Geometry: final body of the model. Coordinates: model frame, mm. A direction names the side the tool comes from. Give positions to 0.01 mm unless a question says otherwise; leave off trailing zeros. Order: outer loops, then holes, each group sorted by start corner. A loop starts at its lowest first (then second) coordinate and runs counter-clockwise, first axis right, second up. Notation, with made-up numbers: M 75.5,-40 L 130.5,-40 A24 ccw 130.5,-12 Z; hole C 54,79 d3. An arc over 180 degrees is marked long. Use CSV: the item, a comma, the result in double quotes.
```python
from build123d import *

# Parameters (mm, degrees)
PAD_DEPTH    = 12
SKETCH001_W  = 160
SKETCH001_H  = 100
PAD001_DEPTH = 10
SKETCH002_R  = 2
POCKET_DEPTH = 22.001


with BuildPart() as part:
    # Sketch → Pad (new body)
    with BuildSketch(Plane.XY):
        Polygon((-50, 340), (50, 340), (50, 100), (80, 100), (80, 0), (50, 0), (50, -11), (-50, -11), (-50, 0), (-80, 0), (-80, 100), (-50, 100), align=None)
    extrude(amount=PAD_DEPTH)

    # Sketch001 (on Face14 of Pad) → Pad001 (join)
    with BuildSketch(Plane.XY.offset(12)):
        with Locations((0, 50)):
            Rectangle(SKETCH001_W, SKETCH001_H)
    extrude(amount=PAD001_DEPTH)

    # Sketch002 (on Face18 of Pad001) → Pocket (cut, through all)
    with BuildSketch(Plane.XY.offset(22)):
        with Locations((-69.908607, 88.239746)):
            Circle(SKETCH002_R)
        with Locations((69.908607, 88.239746)):
            Circle(SKETCH002_R)
        with Locations((69.908607, 10.851752)):
            Circle(SKETCH002_R)
        with Locations((-69.908607, 10.851752)):
            Circle(SKETCH002_R)
    extrude(amount=-POCKET_DEPTH, mode=Mode.SUBTRACT)


solid = part.part
```
1. Section A-A, the plane x = -46. Return the cut outline in (y, z), plus the area to 3 significant figures.
Answer:
outline,"M -11,0 L 340,0 L 340,12 L 100,12 L 100,22 L 0,22 L 0,12 L -11,12 Z"
area,"5,210 mm2"
2. Section B-B, the plane z = 3.25. Return the cut outline in (x, y), plus the area to 3 significant figures.
Answer:
outline,"M -80,0 L -50,0 L -50,-11 L 50,-11 L 50,0 L 80,0 L 80,100 L 50,100 L 50,340 L -50,340 L -50,100 L -80,100 Z; hole C -69.91,10.85 d4; hole C -69.91,88.24 d4; hole C 69.91,10.85 d4; hole C 69.91,88.24 d4"
area,"41,000 mm2"
3. Section C-C, the plane y = 225. Return the cut outline in (x, z), plus the area to 3 significant figures.
Answer:
outline,"M -50,0 L 50,0 L 50,12 L -50,12 Z"
area,"1,200 mm2"
4. Section D-D, the plane x = -62.5. Return the cut outline in (y, z).
Answer:
outline,"M 0,0 L 100,0 L 100,22 L 0,22 Z"
5. Line query: line 1 (Y direction, x = 67, z = 4); line 2 (Z direction, x = 39.5, y = 182); line 3 (X direction, y = 167, z = 1). Output: solid intervals per line, ascending.
Answer:
line 1,"0 to 100"
line 2,"0 to 12"
line 3,"-50 to 50"
6. Pin query (flat end, axial travel): pin 1 Ø9 at (y, z) = (-6.5, 8.5) entering from -X; pin 2 Ø12 at (x, y) = (19, 250) entering from +Z; pin 3 Ø3 at (x, y) = (-69.91, 88.24) entering from +Z; pin 4 Ø4 at (x, z) = (50.5, 6.5) entering from -Y. Return the tip coordinate at first contact, or that it passes through.
Answer:
pin 1,"x = -50"
pin 2,"z = 12"
pin 3,"through"
pin 4,"y = -11"
7. Reachability of faces 1 (the face through (50, -5, 6)), 2 (the face through (1, -5, 12)), 3 (the face through (-50, 218, 6)), 4 (the face through (-50, -6, 6)) from +Z, -Z, +X, -X, +Y, -Y: full face, straight path, thin tool, end or side. Return the list, or none.
Answer:
face 1,"+Z, -Z, +X, -Y"
face 2,"+Z, +X, -X, -Y"
face 3,"+Z, -Z, -X, +Y"
face 4,"+Z, -Z, -X, -Y"
